Check sheet for the modelled part. Datum: model origin and axes. Units: mm. Face numbers are marked on the shaded views. A direction names the side the tool comes from. Coordinates: 2 decimals unless noted, no trailing zeros. Order: outer loops, then holes, each group sorted by start corner. A loop starts at its lowest first (then second) coordinate and runs counter-clockwise, first axis right, second up.
1. Cross-section at C-C (y = -49.5). Enter the section's corners in (x, z) (3 decimals).
2. Cross-section at B-B (x = 65). Enter the section's corners in (y, z) (1 decimal), then the cut area to 3 significant figures.
3. Cross-section at A-A (z = 5). Enter the section's corners in (x, y) (3 decimals).
4. Thickness scan on line 1 (X direction, y = 35.5, z = 3) (3 decimals); line 2 (Y direction, x = -20.5, z = 10); line 3 (Y direction, x = 41.5, z = 56). Record the ranges inside material, lowest first.
5. Draft check along X on the marked faces 5, 6 and 7. Enter one of: released by +X, released by -X, zero draft, split by the parting line, or undercut.
6. Gauge pin test, flat ends, axial feed: pin 1 Ø11 at (y, z) = (-19, 12.5) entering from +X (3 decimals); pin 2 Ø5 at (x, y) = (49.5, 28) entering from +Z; pin 3 Ø8.5 at (y, z) = (19, 19.5) entering from -X (3 decimals); pin 4 Ø6 at (y, z) = (-18, 29.5) entering from +X. Record the tip position at first contact, or that the pin passes through.
7. Set-up check for the marked faces 1, 2, 3 and 4: record each of +Z, -Z, +X, -X, +Y, -Y from which the full face is reachable in a straight line by a thin tool's end or side.
```python
from build123d import *

# Parameters (mm, degrees)
F1_DEPTH = 63.5
F0_W     = 25.4
F0_H     = 19.05
F2_DEPTH = 25.4
F3_DEPTH = 7.9375
F5_R     = 6.35


# Not quite as in the source:
# - a feature names something its author has since deleted; it is built from what else it names


with BuildPart() as f1:
    # F0 (on Front) → F1 (new body, symmetric)
    with BuildSketch(Plane.XZ):
        Polygon((-41.275, 9.525), (-41.275, -9.525), (41.275, -9.525), (41.275, 9.525), (22.225, 9.525), align=None)
    extrude(amount=F1_DEPTH, both=True)

    # F0 (on Front) → F2 (join, symmetric)
    with BuildSketch(Plane.XZ):
        with BuildLine():
            Line((22.225, 9.525), (41.275, 9.525))
            Line((41.275, 9.525), (41.275, 27.0002))
            ThreePointArc((41.275, 27.0002), (45.9246798487, 38.2255201513), (57.15, 42.8752))
            Line((57.15, 42.8752), (60.325, 42.8752))
            Line((60.325, 42.8752), (60.325, 61.9252))
            Line((60.325, 61.9252), (57.15, 61.9252))
            ThreePointArc((57.15, 61.9252), (32.4542956671, 51.6959043329), (22.225, 27.0002))
            Line((22.225, 27.0002), (22.225, 9.525))
        make_face()
        with Locations((73.025, 52.4002)):
            Rectangle(F0_W, F0_H)
    extrude(amount=F2_DEPTH, both=True)

    # F0 (on Front) → F3 (join, symmetric)
    with BuildSketch(Plane.XZ):
        with BuildLine():
            add(Edge.make_bspline(
                [(-41.275, 9.525), (-41.515853256, 47.6718097925), (16.0763282329, 62.4862834811), (57.15, 61.9252)],
                knots=[0, 0, 0, 0, 111.5045361635, 111.5045361635, 111.5045361635, 111.5045361635], degree=3))
            Line((-41.275, 9.525), (22.225, 9.525))
            Line((22.225, 9.525), (22.225, 27.0002))
            ThreePointArc((22.225, 27.0002), (32.4542956671, 51.6959043329), (57.15, 61.9252))
        make_face()
    extrude(amount=F3_DEPTH, both=True)

    # F0 (on Front) → F4 (revolve)
    with BuildSketch(Plane.XZ):
        Polygon((85.725, 66.675), (85.725, 61.9252), (85.725, 42.8752), (85.725, 38.1), (111.125, 38.1), (111.125, 66.675), align=None)
    revolve(axis=Axis((85.725, 0, 52.3875), (0, 0, 1)))

    # F5
    f5_edges = [f1.edges().sort_by_distance(p)[0] for p in [
        (-41.275, -63.5, 0),
        (41.275, -63.5, 0),
        (41.275, 63.5, 0),
        (-41.275, 63.5, 0),
    ]]
    fillet(f5_edges, radius=F5_R)


solid = f1.part
```
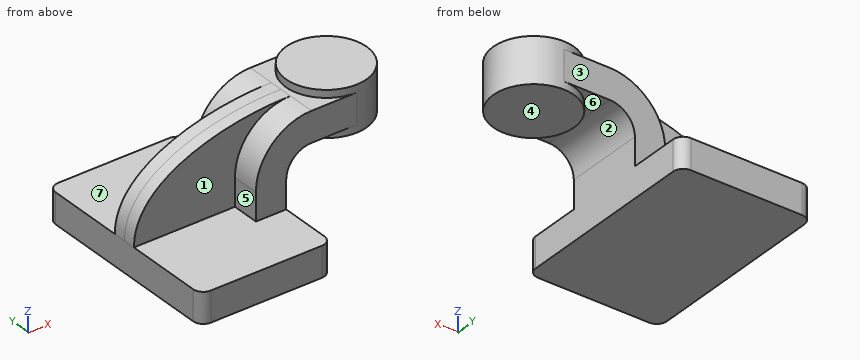
Data:
1. outline: (-41.275, -9.525) - (41.275, -9.525) - (41.275, 9.525) - (-41.275, 9.525) - close
2. outline: (-25.4, 42.9) - (-14.7, 42.9) - (-14.7, 38.1) - (14.7, 38.1) - (14.7, 42.9) - (25.4, 42.9) - (25.4, 61.9) - (14.7, 61.9) - (14.7, 66.7) - (-14.7, 66.7) - (-14.7, 61.9) - (-25.4, 61.9) - close
2. area: 1,250 mm2
3. outline: (-41.275, -57.15) arc R6.35 ccw to (-34.925, -63.5) - (34.925, -63.5) arc R6.35 ccw to (41.275, -57.15) - (41.275, 57.15) arc R6.35 ccw to (34.925, 63.5) - (-34.925, 63.5) arc R6.35 ccw to (-41.275, 57.15) - close
4. line 1: x = -41.275 to 41.275
4. line 2: y = -7.94 to 7.94
4. line 3: y = -25.4 to 25.4
5. face 5: released by -X
5. face 6: undercut
5. face 7: zero draft
6. pin 1: stops at x = 41.275
6. pin 2: passes through
6. pin 3: stops at x = 22.225
6. pin 4: stops at x = 42.26
7. face 1: +Z, -X, -Y
7. face 2: -Z, +Y, -Y
7. face 3: +Z, +X, -X, +Y
7. face 4: -Z, +X, +Y, -Y
